```python
from build123d import *

# Parameters (mm, degrees)
F0_W     = 364.33125
F0_H     = 249.2375
F1_DEPTH = 25.4
F2_W     = 331.7875
F2_H     = 206.375
F3_DEPTH = 0.127
F4_R     = 71.318712
F5_DEPTH = 254


with BuildPart() as f1:
    # F0 (on Front) → F1 (new body)
    with BuildSketch(Plane.XZ):
        Rectangle(F0_W, F0_H)
    extrude(amount=F1_DEPTH)

    # F2 (on face) → F3 (cut)
    with BuildSketch(Plane.XZ.offset(25.4)):
        Rectangle(F2_W, F2_H)
    extrude(amount=-F3_DEPTH, mode=Mode.SUBTRACT)

    # F4 (on face) → F5 (join)
    with BuildSketch(Plane.XZ.offset(25.273)):
        with Locations((11.564023, -30.23188)):
            Circle(F4_R)
    extrude(amount=F5_DEPTH)


solid = f1.part
```
Can you work these out from the model? Positions are in its coordinate system, mm. A direction names the side the tool comes from. Give positions to 0.01 mm unless a question says otherwise; leave off trailing zeros. Order: outer loops, then holes, each group sorted by start corner. A loop starts at its lowest first (then second) coordinate and runs counter-clockwise, first axis right, second up. Notation, with made-up numbers: M 2,84.25 L 29,84.25 A11 ccw 29,105.25 Z; hole C 8.25,3.25 d7. An arc over 180 degrees is marked long. Write item = value, one per line. Start each with the question number.
Q1. Suppose I cut it at D-D (y = -224). Write out the boundary of the cut face in (x, z).
Q2. I need wall thicknesses on probe 1 along Y at (x, z) = (-131, 55); probe 2 along Y at (x, z) = (-127.5, 114); probe 3 along X at (y, z) = (-210, -27.5). Which ranges of each line are inside material? Lowest first, please. Write a range as [from, to].
Q3. Will these pins go through, and if not, where does the flat tip stop? pin 1 Ø2 at (y, z) = (-176.5, 18.5) entering from -X; pin 2 Ø5 at (y, z) = (-240.5, -86) entering from -X; pin 3 Ø1 at (y, z) = (-88.5, -49.5) entering from -X; pin 4 Ø12 at (x, y) = (-71.5, -192) entering from +Z.
Q4. Suppose I cut it at A-A (x = -149.5). Write out the boundary of the cut face in (y, z).
Q5. Suppose I cut it at C-C (z = -71.5). Write out the boundary of the cut face in (x, y), plus the area to 3 significant figures.
Q6. Suppose I cut it at B-B (z = 71). Write out the boundary of the cut face in (x, y).
Q7. For faces 1 (the cylindrical face through (2.28, -150.5, 40.48)), 2 (the flat face through (182.166, -13, -2)), which set-ups out of +Z, -Z, +X, -X, +Y, -Y let a thin tool reach every point of the face, with its end or its side?
Check result:
q1.outline = C 11.56,-30.23 d142.64
q2.probe_1 = [-25.27, 0]
q2.probe_2 = [-25.4, 0]
q2.probe_3 = [-59.7, 82.83]
q3.pin_1 = -41.43
q3.pin_2 = -35.86
q3.pin_3 = -57.24
q3.pin_4 = through
q4.outline = M -25.4,-124.62 L 0,-124.62 L 0,124.62 L -25.4,124.62 L -25.4,103.19 L -25.27,103.19 L -25.27,-103.19 L -25.4,-103.19 Z
q5.outline = M -182.17,-25.4 L -165.89,-25.4 L -165.89,-25.27 L -46.6,-25.27 L -46.6,-279.27 L 69.73,-279.27 L 69.73,-25.27 L 165.89,-25.27 L 165.89,-25.4 L 182.17,-25.4 L 182.17,0 L -182.17,0 Z
q5.area = 38,800 mm2
q6.outline = M -182.17,-25.4 L -165.89,-25.4 L -165.89,-25.27 L 165.89,-25.27 L 165.89,-25.4 L 182.17,-25.4 L 182.17,0 L -182.17,0 Z
q7.face_1 = -Y
q7.face_2 = +Z, -Z, +X, +Y, -Y
